Input: part model. Units: mm. Frame: model coordinates. A direction names the side the tool comes from. Coordinates: 2 decimals unless noted, no trailing zeros. Loops run counter-clockwise (first coordinate to the right, second up) from the corner with the lowest first, then second, coordinate; pieces in that order, holes last.
Item 1: Section A-A on y = -3.5. Return loops of the section in (x, z), and give its area (3 significant figures).
Item 2: Ray query, line 1 along X through (y, z) = (-5.25, -24); line 2 along X through (y, z) = (-13.25, 3); line 3 along Z through (x, y) = (15.5, -23.25). Return the intervals inside material, ascending.
Item 3: Section C-C on y = -8. Return loops of the section in (x, z).
Item 4: Pull-direction query (X, two-part tool) for faces 6 (the cylindrical face through (13.1, -24.1, -18.19)), 7 (the flat face through (16, -13, 20)), 8 (the flat face through (15, -13, -1)), 9 (the cylindrical face through (16.1, -20.8, -30)); classes: released by +X, released by -X, zero draft, split by the parting line, or undercut.
Item 5: Contact query for flat-ended pins moving along their axis: P1, Ø1, axis at x = 17, z = 5, coming from the +Y side; P2, Ø3, axis at y = -23, z = 13, coming from the -X side. Output: stop coordinate, or through.
Item 6: Section D-D on z = -27. Return loops of the section in (x, y).
Item 7: Reachability of faces 1 (the flat face through (11.056, -12.818, -11.077)), 2 (the flat face through (7, -13, -23)), 3 (the flat face through (20, -25, -6)), 4 (the flat face through (10.57, -12.32, -19.31)), 5 (the flat face through (15.4, 0, -1.5)) from +Z, -Z, +X, -X, +Y, -Y: full face, straight path, thin tool, end or side. Return the list, or none.
Item 8: Section B-B on z = 12. Return loops of the section in (x, y), and give its area (3 significant figures).
```python
from build123d import *

# Parameters (mm, degrees)
BOSS_EXTRUDE2_DEPTH = 26
SHELL1_T            = -1
FILLET1_R           = 14
BOSS_EXTRUDE3_REACH = 52.259
FILLET2_R           = 14
SKETCH8_W           = 10.5
SKETCH8_H           = 3
BOSS_EXTRUDE4_DEPTH = 1
SKETCH4_R           = 2
CUT_EXTRUDE1_DEPTH  = 9
BOSS_EXTRUDE5_REACH = 52.259
SKETCH7_R           = 2.4
CUT_EXTRUDE2_DEPTH  = 4.7625
FILLET5_R           = 2


with BuildPart() as part:
    # Sketch2 → Boss-Extrude2 (new body)
    with BuildSketch(Plane.XZ):
        Polygon((7, -12.183821406), (7, -35), (25, -35), (25, 20), (7, 20), (7, 10.183821406), (15, 8), (15, -10), align=None)
    extrude(amount=BOSS_EXTRUDE2_DEPTH)

    # Shell1
    shell1_openings = [part.faces().sort_by_distance(p)[0] for p in [
        (17.00255576, 0, -8.766773004),
    ]]
    offset(amount=SHELL1_T, openings=shell1_openings, kind=Kind.INTERSECTION)

    # Fillet1
    fillet1_edges = [part.edges().sort_by_distance(p)[0] for p in [
        (16, -25, -34),
    ]]
    fillet(fillet1_edges, radius=FILLET1_R)

    # Sketch3 → Boss-Extrude3 (add, up to next)
    with BuildSketch(Plane(origin=(0, 0, 0), x_dir=(1, 0, 0), z_dir=(0, 1, 0)), mode=Mode.PRIVATE) as boss_extrude3_sk1:
        Polygon((13.5, 11.446055541), (8, 12.947432757), (8, 20), (13.5, 18.526279442), align=None)
    boss_extrude3_tool1 = extrude(boss_extrude3_sk1.sketch, amount=-BOSS_EXTRUDE3_REACH, mode=Mode.PRIVATE) - part.part
    # Sketch3 → Boss-Extrude3 (add, up to next)
    with BuildSketch(Plane(origin=(0, 0, 0), x_dir=(1, 0, 0), z_dir=(0, 1, 0)), mode=Mode.PRIVATE) as boss_extrude3_sk2:
        Polygon((13.5, -9.446055541), (8, -10.947432757), (8, -19), (13.5, -19), align=None)
    boss_extrude3_tool2 = extrude(boss_extrude3_sk2.sketch, amount=-BOSS_EXTRUDE3_REACH, mode=Mode.PRIVATE) - part.part
    add(boss_extrude3_tool1.solids().sort_by_distance((10.751794, 0, -15.729457))[0])
    add(boss_extrude3_tool2.solids().sort_by_distance((10.828168, 0, 14.587703))[0])

    # Fillet2
    # the kernel refuses this fillet: 14 mm, written as the material it adds along each edge
    with BuildSketch(Plane(origin=(24, 0, 19), x_dir=(0, 0, -1), z_dir=(0, -1, 0))) as fillet2_piece_1:
        with BuildLine():
            CenterArc((13.555441712, -14), FILLET2_R, 90, 75.522487814)
            Line((0, -10.5), (-0.271108834, -10.43))
            ThreePointArc((-0.271108834, -10.43), (-0.28, -5.25), (-0.28, 0))
            Line((-0.28, 0), (0, 0.28))
            Line((0, 0.28), (13.555441712, 0.28))
            Line((13.555441712, 0.28), (13.555441712, 0))
        make_face()
    extrude(amount=25)

    # Sketch8 → Boss-Extrude4 (add)
    with BuildSketch(Plane(origin=(0, 0, 0), x_dir=(1, 0, 0), z_dir=(0, 1, 0))):
        with Locations((18.75, 17.026279442)):
            Rectangle(SKETCH8_W, SKETCH8_H)
    extrude(amount=-BOSS_EXTRUDE4_DEPTH)

    # Sketch4 → Cut-Extrude1 (cut)
    with BuildSketch(Plane.ZY.offset(-7)):
        with Locations((-15, -23)):
            Circle(SKETCH4_R)
        with Locations((13, -23)):
            Circle(SKETCH4_R)
    extrude(amount=-CUT_EXTRUDE1_DEPTH, mode=Mode.SUBTRACT)

    # Sketch9 → Boss-Extrude5 (add, up to next)
    with BuildSketch(Plane(origin=(0, 0, 0), x_dir=(1, 0, 0), z_dir=(0, 1, 0)), mode=Mode.PRIVATE) as boss_extrude5_sk1:
        with BuildLine():
            Line((13.5, -15), (15.5, -15))
            Line((15.5, -15), (24, -4.870094463))
            Line((24, -4.870094463), (24, -5.444558288))
            ThreePointArc((24, -5.444558288), (21.067971811, -14.017772388), (13.5, -19))
            Line((13.5, -19), (13.5, -15))
        make_face()
    boss_extrude5_tool1 = extrude(boss_extrude5_sk1.sketch, amount=-BOSS_EXTRUDE5_REACH, mode=Mode.PRIVATE) - part.part
    add(boss_extrude5_tool1.solids().sort_by_distance((18.990726, 0, 13.031002))[0])

    # Sketch7 → Cut-Extrude2 (cut)
    with BuildSketch(Plane(origin=(0, 0, 0), x_dir=(1, 0, 0), z_dir=(0, 1, 0))):
        with Locations(Location((20.5, -15.5, 0), (0, 0, 270))):
            Circle(SKETCH7_R)
    extrude(amount=-CUT_EXTRUDE2_DEPTH, mode=Mode.SUBTRACT)

    # Fillet5
    fillet5_edges = [part.edges().sort_by_distance(p)[0] for p in [
        (8, -12.5, -20),
        (13.5, -13, -18.526279442),
    ]]
    fillet(fillet5_edges, radius=FILLET5_R)


solid = part.part
```
Results found:
1. outline: (7, -35) - (25, -35) - (25, 20) - (7, 20) - (7, 10.18) - (15, 8) - (15, -10) - (7, -12.18) - close; hole (8, -34) - (24, -34) - (24, 4.87) - (15.5, 15) - (13.5, 15) - (13.5, 9.45) - (16, 8.76) - (16, -10.76) - (13.5, -11.45) - (13.5, -16.99) arc R2 cw to (12.02, -18.92) - (9.48, -19.6) arc R2 ccw to (8, -21.53) - close; hole circle Ø4.8 at (20.5, 15.5)
1. area: 308 mm2
2. line 1: x = 7 to 8, 24 to 25
2. line 2: x = 15 to 16, 24 to 25
2. line 3: z = -35 to -26.78, -10.9 to 8.9, 15 to 20
3. outline: (7, -35) - (25, -35) - (25, 20) - (7, 20) - (7, 10.18) - (15, 8) - (15, -10) - (7, -12.18) - close; hole (8, -34) - (24, -34) - (24, 4.87) - (15.5, 15) - (13.5, 15) - (13.5, 9.45) - (16, 8.76) - (16, -10.76) - (13.5, -11.45) - (13.5, -16.99) arc R2 cw to (12.02, -18.92) - (9.48, -19.6) arc R2 ccw to (8, -21.53) - close
4. face 6: undercut
4. face 7: zero draft
4. face 8: released by -X
4. face 9: undercut
5. P1: stops at y = -25
5. P2: stops at x = 15.92
6. outline: (7, -26) - (25, -26) - (25, 0) - (24, 0) - (24, -23.12) - (8, -23.12) - (8, 0) - (7, 0) - close
7. face 1: -X, +Y, -Y
7. face 2: +Z, -Z, -X, +Y, -Y
7. face 3: none
7. face 4: +Y
7. face 5: +Z, -Z, +X, -X, +Y
8. outline: (7, -26) - (25, -26) - (25, 0) - (18.02, 0) - (18.02, -25) - (13.5, -25) - (13.5, -24.73) - (7, -24.73) - close; (7, -21.27) - (13.5, -21.27) - (13.5, 0) - (7, 0) - close
8. area: 333 mm2
